Can you work these out from the model? Positions are in its coordinate system, mm. Face numbers are marked on the shaded views. A direction names the side the tool comes from. Coordinates: 2 decimals unless noted, no trailing zeros. Order: outer loops, then holes, each group sorted by start corner. A loop starts at its lowest first (then second) coordinate and runs counter-clockwise, first axis right, second up. Notation, with made-up numbers: (84.5, 66) -> (110.5, 66) arc R34 cw to (110.5, 101) -> close; hole circle Ø4 at (76, 83.5). An arc over 180 degrees is marked (long way). Answer in a Markdown table with one row per item.
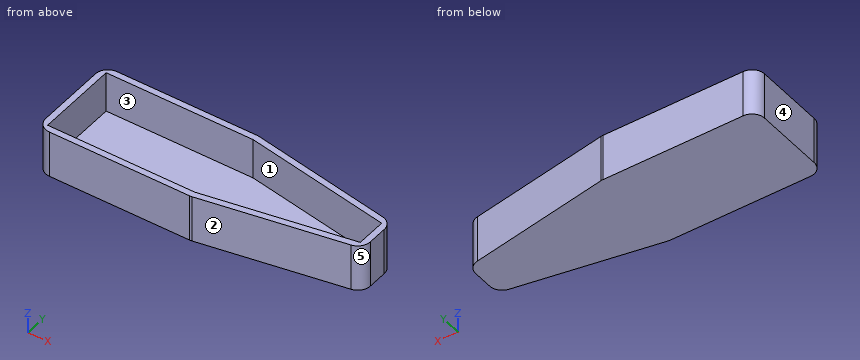
```python
from build123d import *

# Parameters (mm, degrees)
F1_DEPTH    = 8.255
F2_T        = 2.54
F3_T1_DEPTH = 40.3429500211
F3_T3_DEPTH = 21.284150325
F3_T5_DEPTH = 44.45


# Not quite as in the source:
# - a fillet or chamfer that OpenCascade refuses, or shapes differently, is made with other operations: its cross-section is extruded or revolved along the edge and cut away or added


with BuildPart() as f1:
    # F0 (on Top) → F1 (new body, symmetric)
    with BuildSketch(Plane.XY):
        Polygon((0, 16.7005), (-59.7916, 16.7005), (-59.7916, -16.7005), (0, -16.7005), (59.7916, -6.1001079157), (59.7916, 6.1001079157), align=None)
    extrude(amount=F1_DEPTH, both=True)

    # F2
    f2_openings = [f1.faces().sort_by_distance(p)[0] for p in [
        (-7.518342, 0, 8.255),
    ]]
    offset(amount=F2_T, openings=f2_openings, kind=Kind.INTERSECTION)

    # F3: fillet of radius 5.08 on 6 edges, made by hand

    # F3_s2 → F3_t1 (cut)
    with BuildSketch(Plane.XY.offset(-21.4414750105)):
        with BuildLine():
            ThreePointArc((58.1383992054, 8.9728112312), (61.1446283818, 7.2343585343), (62.3316, 3.9708129136))
            Line((62.3316, 3.9708129136), (62.3316, 8.2294029178))
            Line((62.3316, 8.2294029178), (58.1383992054, 8.9728112312))
        make_face()
        with BuildLine():
            ThreePointArc((62.3316, -3.9708129136), (61.1446283818, -7.2343585343), (58.1383992054, -8.9728112312))
            Line((58.1383992054, -8.9728112312), (62.3316, -8.2294029178))
            Line((62.3316, -8.2294029178), (62.3316, -3.9708129136))
        make_face()
    extrude(amount=F3_T1_DEPTH, mode=Mode.SUBTRACT)

    # F3_s4 → F3_t3 (cut)
    with BuildSketch(Plane.XY.offset(-11.9120751625)):
        with BuildLine():
            ThreePointArc((0.6633841729, 19.1624983176), (0.2216964966, 19.2209620072), (-0.2234150325, 19.2405))
            Line((-0.2234150325, 19.2405), (0.2234150325, 19.2405))
            Line((0.2234150325, 19.2405), (0.6633841729, 19.1624983176))
        make_face()
        with BuildLine():
            ThreePointArc((0.6633841729, -19.1624983176), (0.2216964966, -19.2209620072), (-0.2234150325, -19.2405))
            Line((-0.2234150325, -19.2405), (0.2234150325, -19.2405))
            Line((0.2234150325, -19.2405), (0.6633841729, -19.1624983176))
        make_face()
    extrude(amount=F3_T3_DEPTH, mode=Mode.SUBTRACT)

    # F3_s6 → F3_t5 (cut)
    with BuildSketch(Plane.XY.offset(-23.495)):
        with BuildLine():
            ThreePointArc((-57.2516, -19.2405), (-60.8437024484, -17.7526024484), (-62.3316, -14.1605))
            Line((-62.3316, -14.1605), (-62.3316, -19.2405))
            Line((-62.3316, -19.2405), (-57.2516, -19.2405))
        make_face()
        with BuildLine():
            ThreePointArc((-62.3316, 14.1605), (-60.8437024484, 17.7526024484), (-57.2516, 19.2405))
            Line((-57.2516, 19.2405), (-62.3316, 19.2405))
            Line((-62.3316, 19.2405), (-62.3316, 14.1605))
        make_face()
    extrude(amount=F3_T5_DEPTH, mode=Mode.SUBTRACT)


solid = f1.part
```
(1) Suppose I cut it at C-C (y = 12). Please give me the cut outline in (x, z) (3 decimals).
Response values:
| item | result |
|---|---|
| outline | (-62.332, -10.795) -> (41.064, -10.795) -> (41.064, 8.255) -> (26.513, 8.255) -> (26.513, -8.255) -> (-59.792, -8.255) -> (-59.792, 8.255) -> (-62.332, 8.255) -> close |
(2) I need wall thicknesses on line 1 (Y direction, x = -9, z = 3); line 2 (X direction, y = -2, z = -8); line 3 (Z direction, x = 27, y = -5.5) (3 decimals). Which ranges of each line are inside material? Lowest first, please. Write a range as [from, to].
Response values:
| item | result |
|---|---|
| line 1 | [-19.24, -16.7], [16.7, 19.24] |
| line 2 | [-62.33, -59.79], [59.79, 62.33] |
| line 3 | [-10.795, -8.255] |
(3) On a 3-axis mill with a long thin cutter (end or side, diameter ignored), from which of +Z, -Z, +X, -X, +Y, -Y can I reach the whole of each face in a straight line? I mean the marked faces 1 and 2. Say none if no direction works.
Response values:
| item | result |
|---|---|
| face 1 | +Z |
| face 2 | +Z, -Z, +X, -Y |
(4) Suppose I cut it at B-B (x = -22). Please give me the cut outline in (y, z) (1 decimal).
Response values:
| item | result |
|---|---|
| outline | (-19.2, -10.8) -> (19.2, -10.8) -> (19.2, 8.3) -> (16.7, 8.3) -> (16.7, -8.3) -> (-16.7, -8.3) -> (-16.7, 8.3) -> (-19.2, 8.3) -> close |
(5) Will these pins go through, and if not, where does the flat tip stop? pin 1 Ø1.5 at (x, y) = (-21, 9.5) entering from +Z (3 decimals); pin 2 Ø8 at (x, z) = (46, 4.5) entering from -Y; pin 3 Ø1.5 at (x, z) = (8.5, -5) entering from +Y; pin 4 Ø6 at (y, z) = (-7, -2.5) entering from +X.
Response values:
| item | result |
|---|---|
| pin 1 | z = -8.255 |
| pin 2 | y = -11.83 |
| pin 3 | y = 17.91 |
| pin 4 | x = 62.33 |
(6) We'd pull the mould along Y, two halves only. Please class the marked faces 3, 4 and 5: +Y half, -Y half, draft (parallel to the pull), parting line (faces both ways), or undercut.
Response values:
| item | result |
|---|---|
| face 3 | undercut |
| face 4 | draft |
| face 5 | -Y half |
(7) Suppose I cut it at A-A (z = -4.25). Please give me the cut outline in (x, y), and give its area (3 significant figures).
Response values:
| item | result |
|---|---|
| outline | (-62.33, -14.16) arc R5.08 ccw to (-57.25, -19.24) -> (-0.22, -19.24) arc R5.08 ccw to (0.66, -19.16) -> (58.14, -8.97) arc R5.08 ccw to (62.33, -3.97) -> (62.33, 3.97) arc R5.08 ccw to (58.14, 8.97) -> (0.66, 19.16) arc R5.08 ccw to (-0.22, 19.24) -> (-57.25, 19.24) arc R5.08 ccw to (-62.33, 14.16) -> close; hole (-59.79, -16.7) -> (0, -16.7) -> (59.79, -6.1) -> (59.79, 6.1) -> (0, 16.7) -> (-59.79, 16.7) -> close |
| area | 735 mm2 |
